Input: dimensioned drawing with shaded views. Units: mm. Origin: part minimum x, y, z. A direction names the side the tool comes from. Coordinates: 2 decimals unless noted, no trailing zeros. Order: outer loops, then holes, each group sorted by start corner. A loop starts at its lowest first (then second) coordinate and runs counter-clockwise, first axis right, second up. Notation, with made-up numbers: (-31.5, -27) -> (10.5, -27) arc R37 ccw to (10.5, 12) -> close; hole circle Ø2 at (63, 23.25). An arc over 180 degrees is marked (long way). Write item = value, one per line. Start each with the question number.
Item 1: Section query D-D (z = 56.5). Output: boundary loops of the cut face in (x, y), then the cut area to 3 significant figures.
Item 2: Mould query, pull axis X, two halves, no side actions, for the marked faces 4, 5, 6 and 7. Classes: released by +X, released by -X, zero draft, split by the parting line, or undercut.
Item 3: Section query A-A (z = 8). Output: boundary loops of the cut face in (x, y).
Item 4: Section query C-C (y = 78). Output: boundary loops of the cut face in (x, z).
Item 5: Ray query, line 1 along Y through (x, z) = (50, 7); line 2 along X through (y, z) = (41.5, 33.5); line 3 along Z through (x, y) = (5, 43.5). Return the intervals inside material, ascending. Write a range as [from, to].
Item 6: Set-up query: the marked faces 1, 2 and 3. Return all of +Z, -Z, +X, -X, +Y, -Y with unobstructed straight access to the full face (end or side cutting, diameter ignored); none if empty.
Item 7: Contact query for a flat-ended pin moving along its axis: pin 1 (10.5 mm diameter, centred on x = 6, y = 60.5, fed in from +Z). Output: stop coordinate, or through.
Item 8: Section query B-B (x = 58.5). Output: boundary loops of the cut face in (y, z).
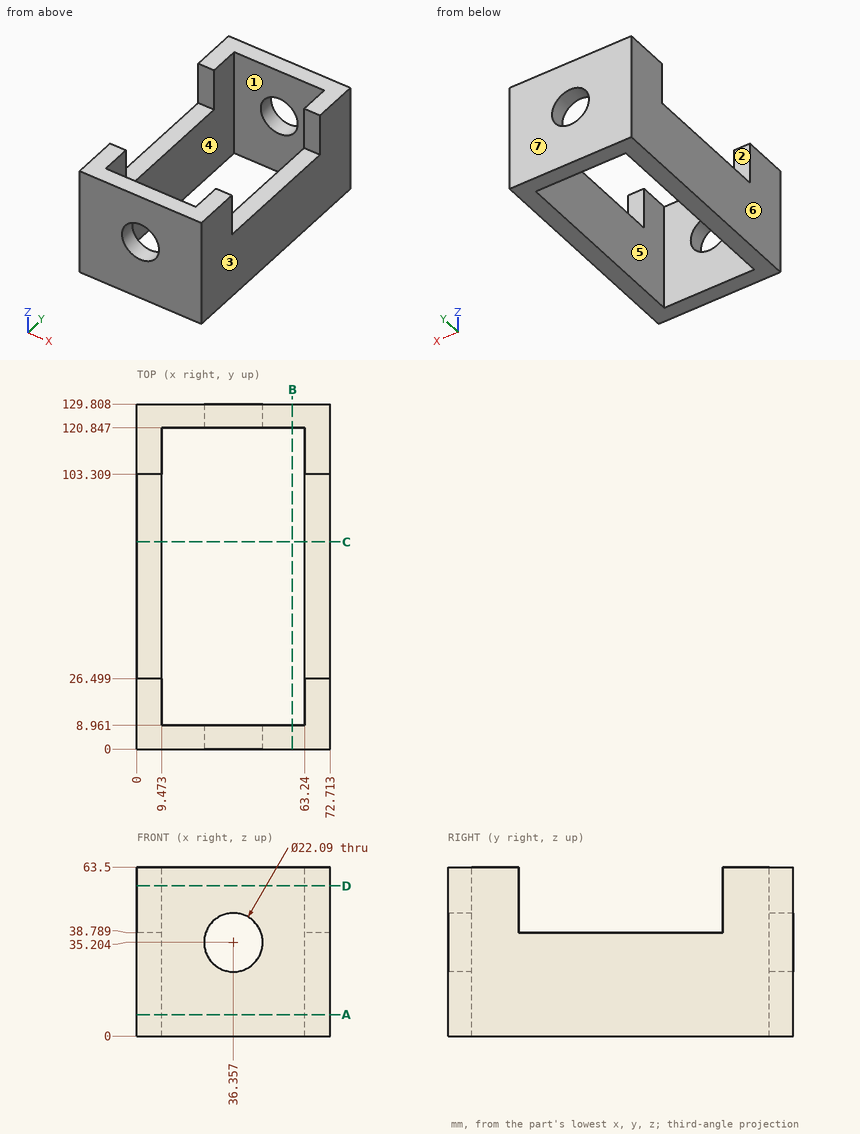
Computed:
q1.outline = (0, 0) -> (72.71, 0) -> (72.71, 26.5) -> (63.24, 26.5) -> (63.24, 8.96) -> (9.47, 8.96) -> (9.47, 26.5) -> (0, 26.5) -> close; (0, 103.31) -> (9.47, 103.31) -> (9.47, 120.85) -> (63.24, 120.85) -> (63.24, 103.31) -> (72.71, 103.31) -> (72.71, 129.81) -> (0, 129.81) -> close
q1.area = 1,970 mm^2
q2.face_4 = undercut
q2.face_5 = undercut
q2.face_6 = released by -X
q2.face_7 = zero draft
q3.outline = (0, 0) -> (72.71, 0) -> (72.71, 129.81) -> (0, 129.81) -> close; hole (9.47, 8.96) -> (63.24, 8.96) -> (63.24, 120.85) -> (9.47, 120.85) -> close
q4.outline = (0, 0) -> (9.47, 0) -> (9.47, 38.79) -> (0, 38.79) -> close; (63.24, 0) -> (72.71, 0) -> (72.71, 38.79) -> (63.24, 38.79) -> close
q5.line_1 = [0, 8.96], [120.85, 129.81]
q5.line_2 = [0, 9.47], [63.24, 72.71]
q5.line_3 = [0, 38.79]
q6.face_1 = +Z, -Z
q6.face_2 = +Z, +X, -X
q6.face_3 = +Z, -Z, +X, +Y, -Y
q7.pin_1 = 38.79
q8.outline = (0, 0) -> (8.96, 0) -> (8.96, 63.5) -> (0, 63.5) -> close; (120.85, 0) -> (129.81, 0) -> (129.81, 63.5) -> (120.85, 63.5) -> close
